```python
from build123d import *

# Parameters (mm, degrees)
F0_W     = 70.42
F0_H     = 45.8
F1_DEPTH = 0.9
F2_W     = 57.288
F2_H     = 38.192
F3_DEPTH = 0.5
F4_W     = 2
F4_H     = 45.8
F5_DEPTH = 0.5


with BuildPart() as f1:
    # F0 (on Top) → F1 (new body)
    with BuildSketch(Plane.XY):
        Rectangle(F0_W, F0_H)
    extrude(amount=F1_DEPTH)

    # F2 (on face) → F3 (cut)
    with BuildSketch(Plane.XY.offset(0.9)):
        with Locations((2.746, 0.004)):
            Rectangle(F2_W, F2_H)
    extrude(amount=-F3_DEPTH, mode=Mode.SUBTRACT)

    # F4 (on face) → F5 (cut)
    with BuildSketch(Plane.XY.offset(0.9)):
        with Locations((-34.21, 0)):
            Rectangle(F4_W, F4_H)
    extrude(amount=-F5_DEPTH, mode=Mode.SUBTRACT)


solid = f1.part
```
Part model, mm, in its own coordinate system. A direction names the side the tool comes from. Give positions to 0.01 mm unless a question says otherwise; leave off trailing zeros. Loops run counter-clockwise (first coordinate to the right, second up) from the corner with the lowest first, then second, coordinate; pieces in that order, holes last. Notation, with made-up numbers: M 37.5,30.5 L 88.5,30.5 A16 ccw 88.5,49.5 Z; hole C -38.75,68 d9. An arc over 180 degrees is marked long. Return JSON: item names as keys, results as strings.
1) Flat gauge pins, fed straight in: pin 1 Ø3 at (x, y) = (-6.5, -9.5) entering from -Z; pin 2 Ø2 at (x, y) = (16, -12) entering from +Z. Where does each tip first touch, or does it go through?
Calculated:
{"pin 1": "stops at z = 0", "pin 2": "stops at z = 0.4"}
2) Drill centre lines: line 1 (Y direction, x = 18, z = 0.65); line 2 (X direction, y = 5.5, z = 0.75); line 3 (X direction, y = 21, z = 0.45). Where is each one in solid material? Low to high.
Calculated:
{"line 1": "y = -22.9 to -19.09, 19.1 to 22.9", "line 2": "x = -33.21 to -25.9, 31.39 to 35.21", "line 3": "x = -33.21 to 35.21"}
3) Saw through at B-B, the plane y = 2. List the corners of the cut face in (x, z).
Calculated:
{"outline": "M -35.21,0 L 35.21,0 L 35.21,0.9 L 31.39,0.9 L 31.39,0.4 L -25.9,0.4 L -25.9,0.9 L -33.21,0.9 L -33.21,0.4 L -35.21,0.4 Z"}
4) Saw through at C-C, the plane x = -9. List the corners of the cut face in (y, z), then the cut area to 3 significant figures.
Calculated:
{"outline": "M -22.9,0 L 22.9,0 L 22.9,0.9 L 19.1,0.9 L 19.1,0.4 L -19.09,0.4 L -19.09,0.9 L -22.9,0.9 Z", "area": "22.1 mm2"}
5) Saw through at A-A, the plane z = 0.6. List the corners of the cut face in (x, y).
Calculated:
{"outline": "M -33.21,-22.9 L 35.21,-22.9 L 35.21,22.9 L -33.21,22.9 Z; hole M -25.9,-19.09 L 31.39,-19.09 L 31.39,19.1 L -25.9,19.1 Z"}
6) 3-axis set-ups, long thin cutter, end or side, ignore diameter. For faces 1 (the face through (-7, 20, 0.9)), 2 (the face through (-34, 0, 0.4)), 3 (the face through (2, 0, 0.4)): which of +Z, -Z, +X, -X, +Y, -Y reach the whole face in a straight line?
Calculated:
{"face 1": "+Z, +X, -X, +Y, -Y", "face 2": "+Z, -X, +Y, -Y", "face 3": "+Z"}
